Could you check a few things on this model? Use its own coordinates, in mm. Face numbers are marked on the shaded views. A direction names the side the tool comes from. Give positions to 0.01 mm unless a question says otherwise; leave off trailing zeros. Order: outer loops, then holes, each group sorted by start corner. A loop starts at its lowest first (then second) coordinate and runs counter-clockwise, first axis right, second up. Notation, with made-up numbers: (-11, -13) -> (46, -13) arc R22 ccw to (46, 25) -> close; hole circle Ø10 at (55, -1.5). An arc over 180 degrees is marked (long way). Use one line per item in the form item = value. Start each with the question number.
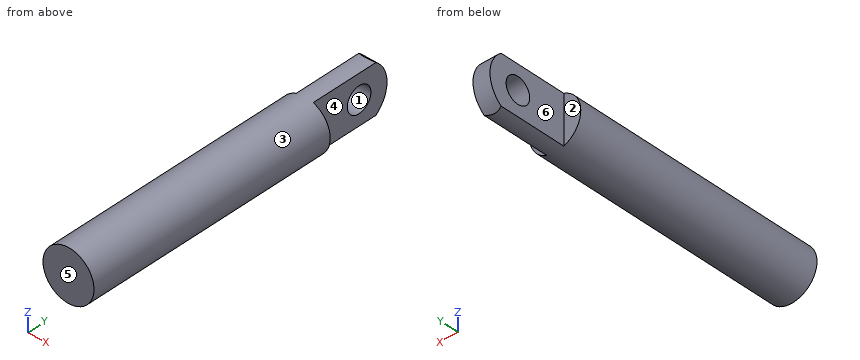
from build123d import *

# Parameters (mm, degrees)
SKETCH1_R               = 3
BOSS_EXTRUDE1_DEPTH     = 30
BOSS_EXTRUDE2_START     = 10
BOSS_EXTRUDE2_DEPTH     = 10
SKETCH2_R               = 1.5
CUT_EXTRUDE1_DEPTH      = 10
CUT_EXTRUDE2_DEPTH      = 31.413812651
CUT_EXTRUDE2_DEPTH_BACK = 31.413812651


with BuildPart() as part:
    # Sketch1 → Boss-Extrude1 (new body)
    with BuildSketch(Plane(origin=(0, 0, 0), x_dir=(1, 0, 0), z_dir=(0, 1, 0))):
        with Locations(Location((0, 0, 0), (0, 0, 270))):
            Circle(SKETCH1_R)
    extrude(amount=-BOSS_EXTRUDE1_DEPTH)

    # Sketch1_3 → Boss-Extrude2 (add)
    with BuildSketch(Plane(origin=(0, 0, 0), x_dir=(1, 0, 0), z_dir=(0, 1, 0)).offset(BOSS_EXTRUDE2_START)):
        with BuildLine():
            ThreePointArc((-1, -2.828427125), (0, -3), (1, -2.828427125))
            Line((1, -2.828427125), (1, 2.828427125))
            ThreePointArc((1, 2.828427125), (0, 3), (-1, 2.828427125))
            Line((-1, 2.828427125), (-1, -2.828427125))
        make_face()
    extrude(amount=-BOSS_EXTRUDE2_DEPTH)

    # Sketch2 → Cut-Extrude1 (cut)
    with BuildSketch(Plane(origin=(1, 0, 0), x_dir=(0, 0, -1), z_dir=(1, 0, 0))):
        with Locations((0, 5.828656685)):
            Circle(SKETCH2_R)
    extrude(amount=-CUT_EXTRUDE1_DEPTH, mode=Mode.SUBTRACT)

    # Sketch3 → Cut-Extrude2 (cut, two sides: drawn at the far end of the back side and taken through both)
    with BuildSketch(Plane(origin=(1, 0, 0), x_dir=(0, 0, -1), z_dir=(1, 0, 0)).offset(-CUT_EXTRUDE2_DEPTH_BACK)):
        with BuildLine():
            Line((3.541708321, 5.828656685), (6.198168723, 5.828656685))
            Line((6.198168723, 5.828656685), (6.198168723, 11.427002628))
            Line((6.198168723, 11.427002628), (-4.798582237, 11.427002628))
            Line((-4.798582237, 11.427002628), (-4.798582237, 5.828656685))
            Line((-4.798582237, 5.828656685), (-3.541708321, 5.828656685))
            ThreePointArc((-3.541708321, 5.828656685), (0, 9.370365006), (3.541708321, 5.828656685))
        make_face()
    extrude(amount=CUT_EXTRUDE2_DEPTH + CUT_EXTRUDE2_DEPTH_BACK, mode=Mode.SUBTRACT)


solid = part.part
(1) We'd pull the mould along Z, two halves only. Please class the marked faces 1, 2 and 3: pulls with the +Z half, pulls with the -Z half, needs draft (parallel to the pull), parting line crosses it, or undercut.
(2) Imagine slicing it at D-D (z = 2). Write out the boundary of the cut face in (x, y).
(3) Imagine slicing it at C-C (y = 1.5). Write out the boundary of the cut face in (x, z), plus the area to 3 significant figures.
(4) Which directions (+Z, -Z, +X, -X, +Y, -Y) give clear straight access to the entire face, cutting with the end or side of a thin tool? Please do the marked faces 4, 5 and 6.
(5) Please list where these lines run through material, in increasing order: probe 1 along Y at (x, z) = (0.25, 0); probe 2 along Z at (x, y) = (1, -10.5); probe 3 along X at (y, z) = (3.5, 2.75).
(6) Imagine slicing it at A-A (z = 0). Write out the boundary of the cut face in (x, y), plus the area to 3 significant figures.
(7) I'm going to push flat-ended pins straight in: pin 1 Ø1.5 at (y, z) = (-21.5, 1) entering from +X; pin 2 Ø1 at (x, z) = (-2, 0.5) entering from +Y; pin 3 Ø1 at (y, z) = (-6.5, -1.5) entering from +X. Where does each tip first touch, or does it pass through?
(8) Imagine slicing it at B-B (x = 0). Write out the boundary of the cut face in (y, z).
Calculated:
q1.face_1 = undercut
q1.face_2 = needs draft
q1.face_3 = parting line crosses it
q2.outline = (-2.24, -30) -> (2.24, -30) -> (2.24, 0) -> (1, 0) -> (1, 8.75) -> (-1, 8.75) -> (-1, 0) -> (-2.24, 0) -> close
q3.outline = (-1, -2.83) arc R3 ccw to (1, -2.83) -> (1, 2.83) arc R3 ccw to (-1, 2.83) -> close
q3.area = 11.8 mm2
q4.face_4 = +Z, -Z, +X, +Y
q4.face_5 = +Z, -Z, +X, -X, -Y
q4.face_6 = +Z, -Z, -X, +Y
q5.probe_1 = -30 to 4.33, 7.33 to 9.37
q5.probe_2 = -2.83 to 2.83
q5.probe_3 = -1 to 1
q6.outline = (-3, -30) -> (3, -30) -> (3, 0) -> (1, 0) -> (1, 4.33) -> (-1, 4.33) -> (-1, 0) -> (-3, 0) -> close; (-1, 7.33) -> (1, 7.33) -> (1, 9.37) -> (-1, 9.37) -> close
q6.area = 193 mm2
q7.pin_1 = 2.99
q7.pin_2 = 0
q7.pin_3 = 2.83
q8.outline = (-30, -3) -> (7.71, -3) arc R3.54 ccw to (7.71, 3) -> (-30, 3) -> close; hole circle Ø3 at (5.83, 0)
